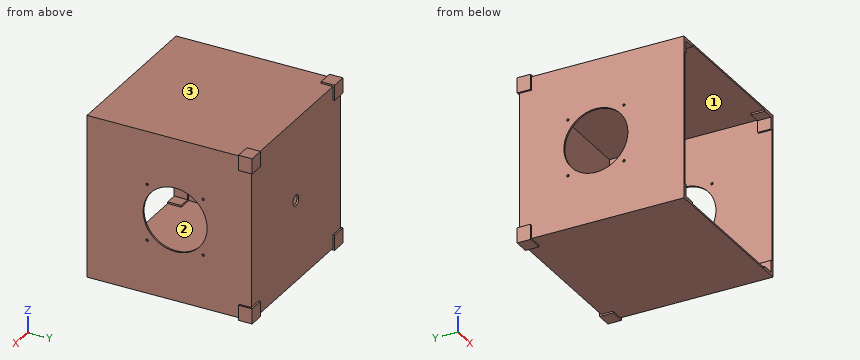
from build123d import *

# Parameters (mm, degrees)
SKETCH1_W               = 304.8
SKETCH1_H               = 304.8
SKETCH1_W_2             = 298.45
SKETCH1_H_2             = 298.45
SKETCH1_R               = 10
BOSS_EXTRUDE1_DEPTH     = 3.175
SKETCH1_3_W             = 304.8
SKETCH1_3_H             = 304.8
SKETCH1_3_W_2           = 298.45
SKETCH1_3_H_2           = 298.45
BOSS_EXTRUDE2_DEPTH     = 307.975
SKETCH3_W               = 25.4
SKETCH3_H               = 25.4
BOSS_EXTRUDE3_DEPTH     = 3.175
BOSS_EXTRUDE4_START     = -22.225
BOSS_EXTRUDE4_DEPTH     = 25.4
CIRPATTERN1_COUNT       = 4
BOSS_EXTRUDE5_DEPTH     = 25.4
CIRPATTERN2_COUNT       = 4
CUT_EXTRUDE1_DEPTH      = 461.385948146
CUT_EXTRUDE1_DEPTH_BACK = 461.385948146
SKETCH6_R               = 60
SKETCH6_R_2             = 2.25


with BuildPart() as part:
    # Sketch1 → Boss-Extrude1 (new body)
    # profile 1 of 2: a face of its own
    with BuildSketch(Plane(origin=(0, 0, 0), x_dir=(1, 0, 0), z_dir=(0, 1, 0))):
        Rectangle(SKETCH1_W, SKETCH1_H)
        Rectangle(SKETCH1_W_2, SKETCH1_H_2, mode=Mode.SUBTRACT)
    # profile 2 of 2: a face of its own
    with BuildSketch(Plane(origin=(0, 0, 0), x_dir=(1, 0, 0), z_dir=(0, 1, 0))):
        Rectangle(SKETCH1_W_2, SKETCH1_H_2)
        with Locations(Location((0, 0, 0), (0, 0, 270))):
            Circle(SKETCH1_R, mode=Mode.SUBTRACT)
    extrude(amount=-BOSS_EXTRUDE1_DEPTH)

    # Sketch1_3 → Boss-Extrude2 (add)
    with BuildSketch(Plane(origin=(0, 0, 0), x_dir=(1, 0, 0), z_dir=(0, 1, 0))):
        Rectangle(SKETCH1_3_W, SKETCH1_3_H)
        Rectangle(SKETCH1_3_W_2, SKETCH1_3_H_2, mode=Mode.SUBTRACT)
    extrude(amount=-BOSS_EXTRUDE2_DEPTH)

    # Sketch3 → Boss-Extrude3 (add)
    with BuildSketch(Plane(origin=(0, 0, 0), x_dir=(1, 0, 0), z_dir=(0, 1, 0))):
        with Locations((-139.7, 139.7)):
            Rectangle(SKETCH3_W, SKETCH3_H)
    boss_extrude3 = extrude(amount=BOSS_EXTRUDE3_DEPTH)

    # Sketch3_3 → Boss-Extrude4 (add)
    with BuildSketch(Plane(origin=(0, 0, 0), x_dir=(1, 0, 0), z_dir=(0, 1, 0)).offset(BOSS_EXTRUDE4_START)):
        Polygon((-152.4, 127), (-152.4, 152.4), (-127, 152.4), (-127, 155.575), (-155.575, 155.575), (-155.575, 127), align=None)
    boss_extrude4 = extrude(amount=BOSS_EXTRUDE4_DEPTH)

    # CirPattern1: Boss-Extrude3, Boss-Extrude4 ×4 about axis
    cirpattern1_axis = Axis((0, 0, 0), (0, 1, 0))
    add([boss_extrude3.rotate(cirpattern1_axis, i * 360 / CIRPATTERN1_COUNT) for i in range(1, CIRPATTERN1_COUNT)])
    add([boss_extrude4.rotate(cirpattern1_axis, i * 360 / CIRPATTERN1_COUNT) for i in range(1, CIRPATTERN1_COUNT)])

    # Sketch5 → Boss-Extrude5 (add)
    with BuildSketch(Plane.XZ.offset(307.975)):
        Polygon((-149.225, 123.825), (-146.05, 123.825), (-146.05, 146.05), (-123.825, 146.05), (-123.825, 149.225), (-149.225, 149.225), align=None)
    boss_extrude5 = extrude(amount=-BOSS_EXTRUDE5_DEPTH)

    # CirPattern2: Boss-Extrude5 ×4 about axis
    cirpattern2_axis = Axis((0, 0, 0), (0, 1, 0))
    for i in range(1, CIRPATTERN2_COUNT):
        add(boss_extrude5.rotate(cirpattern2_axis, i * 360 / CIRPATTERN2_COUNT))

    # Sketch6 → Cut-Extrude1 (cut, two sides: drawn at the far end of the back side and taken through both)
    with BuildSketch(Plane.ZY.offset(-149.225).offset(-CUT_EXTRUDE1_DEPTH_BACK)):
        with Locations(Location((0, -142.875, 0), (0, 0, 180))):
            Circle(SKETCH6_R)
        with Locations(Location((-52.5, -90.375, 0), (0, 0, 180))):
            Circle(SKETCH6_R_2)
        with Locations(Location((52.5, -90.375, 0), (0, 0, 180))):
            Circle(SKETCH6_R_2)
        with Locations(Location((52.5, -195.375, 0), (0, 0, 180))):
            Circle(SKETCH6_R_2)
        with Locations(Location((-52.5, -195.375, 0), (0, 0, 180))):
            Circle(SKETCH6_R_2)
    extrude(amount=CUT_EXTRUDE1_DEPTH + CUT_EXTRUDE1_DEPTH_BACK, mode=Mode.SUBTRACT)


solid = part.part
Read the model definition and answer for the solid it produces. Units are mm, in the model's axes. Face numbers are marked on the shaded views. Coordinates: 2 decimals unless noted, no trailing zeros. Loops run counter-clockwise (first coordinate to the right, second up) from the corner with the lowest first, then second, coordinate; pieces in that order, holes last.
Q1. The part is cut by section B-B on z = 0. Write down the section's boundary in (x, y) (3 decimals).
Q2. Each of these flat-tipped pins is pushed along its axis until it touches: pin 1 Ø10 at (x, z) = (69, 95) entering from +Y; pin 2 Ø1 at (y, z) = (-41.5, 13) entering from -X; pin 3 Ø8.5 at (x, z) = (135.5, 141.5) entering from -Y (3 decimals). Where does it stop, or does it pass through?
Q3. The part is cut by section D-D on z = -91. Write down the section's boundary in (x, y) (3 decimals).
Q4. The part is cut by section A-A on x = 0. Write down the section's boundary in (y, z) (3 decimals).
Q5. Consider probe 1 along Z at (x, y) = (108.5, -33) (3 decimals); probe 2 along Y at (x, z) = (-150, 52) (3 decimals). Determine where each line is inside the solid, lowest interval first.
Q6. The part is cut by section C-C on y = -261. Write down the section's boundary in (x, z) (3 decimals), and give its area (3 significant figures).
Q7. The mould has two halves that part along Y. Classify the marked faces 1, 2 and 3: +Y half, -Y half, draft (parallel to the pull), parting line (faces both ways), or undercut.
Results below:
1. outline: (-152.4, -307.975) - (-149.225, -307.975) - (-149.225, -202.875) - (-152.4, -202.875) - close; (-152.4, -82.875) - (-149.225, -82.875) - (-149.225, -3.175) - (-10, -3.175) - (-10, 0) - (-152.4, 0) - close; (10, -3.175) - (149.225, -3.175) - (149.225, -82.875) - (152.4, -82.875) - (152.4, 0) - (10, 0) - close; (149.225, -307.975) - (152.4, -307.975) - (152.4, -202.875) - (149.225, -202.875) - close
2. pin 1: stops at y = 0
2. pin 2: stops at x = -152.4
2. pin 3: stops at y = -3.175
3. outline: (-152.4, -307.975) - (-149.225, -307.975) - (-149.225, -3.175) - (149.225, -3.175) - (149.225, -307.975) - (152.4, -307.975) - (152.4, 0) - (-152.4, 0) - close
4. outline: (-307.975, -152.4) - (0, -152.4) - (0, -10) - (-3.175, -10) - (-3.175, -149.225) - (-307.975, -149.225) - close; (-307.975, 149.225) - (-3.175, 149.225) - (-3.175, 10) - (0, 10) - (0, 152.4) - (-307.975, 152.4) - close
5. probe 1: z = -152.4 to -149.225, 149.225 to 152.4
5. probe 2: y = -307.975 to -197.569, -193.181 to -172.808, -112.942 to -92.569, -88.181 to 0
6. outline: (-152.4, -152.4) - (152.4, -152.4) - (152.4, 152.4) - (-152.4, 152.4) - close; hole (-149.225, -149.225) - (149.225, -149.225) - (149.225, 149.225) - (-149.225, 149.225) - close
6. area: 3,830 mm2
7. face 1: undercut
7. face 2: undercut
7. face 3: draft
